The model under review builds one solid part; all positions refer to its coordinate system, in mm. A direction names the side the tool comes from. Give positions to 0.01 mm unless a question says otherwise; leave off trailing zeros. Order: outer loops, then holes, each group sorted by start corner. A loop starts at its lowest first (then second) coordinate and runs counter-clockwise, first axis right, second up. Notation, with made-up numbers: (66.5, 49) -> (76.5, 49) arc R25 cw to (76.5, 80) -> close; hole circle Ø6 at (21.25, -39.75). An arc over 180 degrees is marked (long way). Answer as a JSON object with one key per item and string values. Group by question number.
from build123d import *

# Parameters (mm, degrees)
BASE_EXTRUDE_THIN_DEPTH = 152.4
CUT_CNR_DEPTH           = 7.35
CUT_CNR_DEPTH_BACK      = 50.276
HOLE_FLG_D              = 13.462
HOLE_TOP_D              = 13.49375
HOLE_TOP_DEPTH          = 25.4


with BuildPart() as part:
    # Sketch1 → Base-Extrude-Thin (new body)
    with BuildSketch(Plane.XY):
        with BuildLine():
            Line((-228.6, 0), (-6.35, 0))
            ThreePointArc((-6.35, 0), (-1.859871939, -1.859871939), (0, -6.35))
            Line((0, -6.35), (0, -49.276))
            Line((0, -49.276), (6.35, -49.276))
            Line((6.35, -49.276), (6.35, -6.35))
            ThreePointArc((6.35, -6.35), (2.630256121, 2.630256121), (-6.35, 6.35))
            Line((-6.35, 6.35), (-228.6, 6.35))
            Line((-228.6, 6.35), (-228.6, 0))
        make_face()
    extrude(amount=BASE_EXTRUDE_THIN_DEPTH)

    # Sketch2 → Cut cnr (cut, two sides)
    with BuildSketch(Plane(origin=(0, 0, 0), x_dir=(1, 0, 0), z_dir=(0, 1, 0))) as cut_cnr_sk:
        Polygon((-731.624052823, 122.482726079), (-228.6, -69.85), (-12.7, -152.4), (490.324052823, -344.732726079), (105.658600664, -1350.780831726), (-1116.289504982, -883.565379567), align=None)
    extrude(amount=CUT_CNR_DEPTH, mode=Mode.SUBTRACT)
    extrude(cut_cnr_sk.sketch, amount=-CUT_CNR_DEPTH_BACK, mode=Mode.SUBTRACT)

    # Hole-flg (through all)
    with Locations(Plane(origin=(6.35, 0, 0), x_dir=(0, 0, -1), z_dir=(1, 0, 0))):
        with Locations((-130.175, -23.8125), (-31.75, -23.8125)):
            Hole(HOLE_FLG_D / 2)

    # Hole-top
    with Locations(Plane(origin=(0, 6.35, 0), x_dir=(-1, 0, 0), z_dir=(0, 1, 0))):
        with Locations((203.2, 31.75), (133.35, 31.75)):
            Hole(HOLE_TOP_D / 2, depth=HOLE_TOP_DEPTH)


solid = part.part
1. Take a section at A-A on z = 31.75. Give the boundary of the cut face in (x, y), plus the area to 3 significant figures.
2. Take a section at D-D on z = 109.5. Give the boundary of the cut face in (x, y), plus the area to 3 significant figures.
3. Draft analysis for pull direction X (two halves, no side actions). For faces 1 (the flat face through (0, -28, 75)), 2 (the cylindrical face through (-140.09, 3.13, 32.05)), 3 (the flat face through (-86, 1, 0)), state which applies: pulls with the +X half, pulls with the -X half, needs draft (parallel to the pull), parting line crosses it, or undercut.
4. Machinability: for faces 4 (the flat face through (-94, 0, 58)), 5 (the flat face through (6.35, -28, 75)), which of the approach directions +Z, -Z, +X, -X, +Y, -Y give a long, thin tool a straight path to every point of the face, cutting with its end or side? Answer none if there is none.
5. For probe 1 along X at (y, z) = (-21, 77); probe 2 along Y at (x, z) = (4, 31.75), list the stretches that pass through material, from the lowest coordinate up. Write a range as [from, to].
6. Take a section at B-B on y = -27. Give the boundary of the cut face in (x, z), plus the area to 3 significant figures.
7. Take a section at C-C on x = -133.35. Give the boundary of the cut face in (y, z), plus the area to 3 significant figures.
8. For pin 1 (21.5 mm diameter, centred on y = -25, z = 66.5, fed in from -X); pin 2 (2 mm diameter, centred on x = -63.5, z = 82, fed in from -Y); pin 3 (12 mm diameter, centred on y = -23.81, z = 130.18, fed in from +X), all flat-tipped, find the tip position at first contact; note any pin that passes through.
Checks:
{
 "1": {"outline": "(-228.6, 0) -> (-209.95, 0) -> (-209.95, 6.35) -> (-228.6, 6.35) -> close; (-196.45, 0) -> (-140.1, 0) -> (-140.1, 6.35) -> (-196.45, 6.35) -> close; (-126.6, 0) -> (-6.35, 0) arc R6.35 cw to (0, -6.35) -> (0, -17.08) -> (6.35, -17.08) -> (6.35, -6.35) arc R12.7 ccw to (-6.35, 6.35) -> (-126.6, 6.35) -> close; (0, -49.28) -> (6.35, -49.28) -> (6.35, -30.54) -> (0, -30.54) -> close", "area": "1,520 mm2"},
 "2": {"outline": "(-124.9, 0) -> (-6.35, 0) arc R6.35 cw to (0, -6.35) -> (0, -49.28) -> (6.35, -49.28) -> (6.35, -6.35) arc R12.7 ccw to (-6.35, 6.35) -> (-124.9, 6.35) -> close", "area": "1,120 mm2"},
 "3": {"face 1": "pulls with the -X half", "face 2": "undercut", "face 3": "needs draft"},
 "4": {"face 4": "+Z, -Z, -X, -Y", "face 5": "+Z, -Z, +X, +Y, -Y"},
 "5": {"probe 1": "x = [0, 6.35]", "probe 2": "y = [-49.28, -30.54], [-17.08, 1.01]"},
 "6": {"outline": "(0, 0) -> (6.35, 0) -> (6.35, 25.82) -> (0, 25.82) -> close; (0, 37.68) -> (6.35, 37.68) -> (6.35, 124.25) -> (0, 124.25) -> close; (0, 136.1) -> (6.35, 136.1) -> (6.35, 152.4) -> (0, 152.4) -> close", "area": "817 mm2"},
 "7": {"outline": "(0, 0) -> (6.35, 0) -> (6.35, 25) -> (0, 25) -> close; (0, 38.5) -> (6.35, 38.5) -> (6.35, 106.27) -> (0, 106.27) -> close", "area": "589 mm2"},
 "8": {"pin 1": "stops at x = 0", "pin 2": "stops at y = 0", "pin 3": "passes through"}
}
